For this review, take the finished solid that the model builds, in its own axes (mm). Face numbers are marked on the shaded views. A direction names the side the tool comes from. Round coordinates to 2 decimals unless told otherwise and drop trailing zeros. Loops run counter-clockwise (first coordinate to the right, second up) from the corner with the lowest first, then second, coordinate; pieces in that order, holes last.
1) Take a section at C-C (y = -8.5). State the section outline as (x, z) points.
2) Take a section at A-A (x = 0). State the section outline as (y, z) points, then the cut area to 3 significant figures.
3) Take a section at D-D (z = -9). State the section outline as (x, y) points, then the cut area to 3 significant figures.
4) Wall thickness on L1, parallel to X at y = -5.25, z = 0; L2, parallel to Z at x = 0, y = -2.25; L3, parallel to X at y = -2.25, z = 0.25: over which ranges is each line inside the solid? List them lowest first.
5) Take a section at B-B (z = 0). State the section outline as (x, y) points, then the cut area to 3 significant figures.
6) Tool access review of the marked faces 4 and 5: name each direction out of +Z, -Z, +X, -X, +Y, -Y from which nothing blocks a thin tool from reaching the whole face with its end or side.
7) Mouldability with a two-part tool opening along Z and no side actions: class the marked faces 1, 2 and 3 as pulls with the +Z half, pulls with the -Z half, needs draft (parallel to the pull), parting line crosses it, or undercut.
8) Insertion check: pin 1 (5.5 mm diameter, centred on x = 0, z = 0, fed in from -Y); pin 2 (1 mm diameter, centred on x = 4.5, y = -3, fed in from +Z); pin 3 (1.5 mm diameter, centred on x = 4, z = -7, fed in from +Y); pin 4 (3 mm diameter, centred on x = -1, y = -5, fed in from -Z). Each pin has a flat end and moves straight along its axis. Give the tip position at first contact, or say it passes through.
```python
from build123d import *

# Parameters (mm, degrees)
CYLINDER011007_R     = 2.2
CYLINDER011007_DEPTH = 20
CYLINDER011006_R     = 12
CYLINDER011006_DEPTH = 2
CYLINDER011009_R     = 0.5
CYLINDER011009_DEPTH = 7
ARRAY007_COUNT       = 22
CYLINDER011005_R     = 6
CYLINDER011005_DEPTH = 7


with BuildPart() as belt_attach_insert_hole:
    # Cylinder011007 → Cylinder011007 (new body)
    with BuildSketch(Plane.XZ):
        Circle(CYLINDER011007_R)
    extrude(amount=CYLINDER011007_DEPTH)


with BuildPart() as belt_disk:
    # Cylinder011006 → Cylinder011006 (new body)
    with BuildSketch(Plane.XZ.offset(7)):
        Circle(CYLINDER011006_R)
    extrude(amount=CYLINDER011006_DEPTH)


with BuildPart() as belt_pin_array:
    # Cylinder011009 → Cylinder011009 (new body)
    with BuildSketch(Plane(origin=(6, 0, 0), x_dir=(1, 0, 0), z_dir=(0, -1, 0))):
        Circle(CYLINDER011009_R)
    extrude(amount=CYLINDER011009_DEPTH)

    # Array007: belt pin array ×22 about axis
    array007_axis = Axis((0, 0, 0), (0, 1, 0))


with BuildPart() as belt_pin_array_1:
    add(belt_pin_array.part)
    for i in range(1, ARRAY007_COUNT):
        add(belt_pin_array.part.rotate(array007_axis, i * 360 / ARRAY007_COUNT))


with BuildPart() as belt_attach_cut:
    # Cylinder011005 → Cylinder011005 (new body)
    with BuildSketch(Plane.XZ):
        Circle(CYLINDER011005_R)
    extrude(amount=CYLINDER011005_DEPTH)

    # Fusion003: union belt disk, belt pin array
    add(belt_disk.part)
    add(belt_pin_array_1.part)

    # Cut023015009007: cut belt attach insert hole
    add(belt_attach_insert_hole.part, mode=Mode.SUBTRACT)


solid = belt_attach_cut.part
```
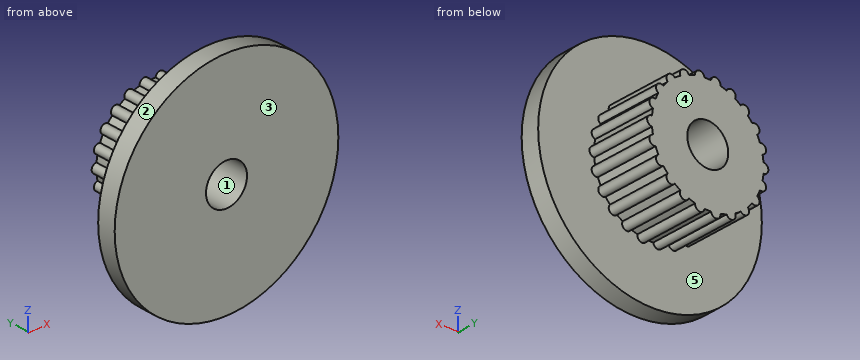
Response:
1. outline: circle Ø24 at (0, 0); hole circle Ø4.4 at (0, 0)
2. outline: (-9, -12) - (-7, -12) - (-7, -6) - (0, -6) - (0, -2.2) - (-9, -2.2) - close; (-9, 2.2) - (0, 2.2) - (0, 6) - (-7, 6) - (-7, 12) - (-9, 12) - close
2. area: 92.4 mm2
3. outline: (-7.94, -9) - (7.94, -9) - (7.94, -7) - (-7.94, -7) - close
3. area: 31.7 mm2
4. L1: x = -6.5 to -2.2, 2.2 to 6.5
4. L2: z = -6 to -2.2, 2.2 to 6
4. L3: x = -6.43 to -2.19, 2.19 to 6.43
5. outline: (-12, -9) - (-2.2, -9) - (-2.2, 0) - (-6.5, 0) - (-6.5, -7) - (-12, -7) - close; (2.2, -9) - (12, -9) - (12, -7) - (6.5, -7) - (6.5, 0) - (2.2, 0) - close
5. area: 99.4 mm2
6. face 4: +Z, -Z, +X, -X, +Y
6. face 5: +Y
7. face 1: undercut
7. face 2: parting line crosses it
7. face 3: needs draft
8. pin 1: stops at y = -9
8. pin 2: stops at z = 5.03
8. pin 3: stops at y = -7
8. pin 4: stops at z = -6.44
